Work out the finished part from the listing and answer in its coordinate system (mm). A direction names the side the tool comes from. Round coordinates to 2 decimals unless told otherwise and drop trailing zeros. Write each loop counter-clockwise with the first axis right and the second up, starting at its lowest first coordinate (ties: lowest second). Pieces come first, ordered by that corner, then holes. Notation, with made-up numbers: (20, 55.5) -> (61, 55.5) arc R27 ccw to (61, 90.5) -> close; hole circle Ø10 at (11, 48). An arc over 180 degrees is marked (long way). One line per item, written item: value.
```python
from build123d import *

# Parameters (mm, degrees)
RESSALTO_EXTRUS_O2_DEPTH = 25
ESBO_O9_R                = 3.75
ESBO_O9_R_2              = 1.65
CORTE_EXTRUS_O1_DEPTH    = 20
FILETE1_R                = 12.5
FILETE2_START            = -1
FILETE2_DEPTH            = 27
FILETE2_2_DEPTH          = 25
ESBO_O10_R               = 1
CORTE_EXTRUS_O2_DEPTH    = 82.160967921
ESBO_O11_R               = 7.5
CORTE_EXTRUS_O3_DEPTH    = 10
FILETE3_R                = 4


with BuildPart() as part:
    # Esboço2 → Ressalto-extrusão2 (new body)
    with BuildSketch(Plane(origin=(0, 0, 0), x_dir=(0, 0, -1), z_dir=(1, 0, 0))):
        Polygon((-5, 0), (0, 0), (5, 0), (69.5, -5.643018797), (69.5, -33.643018797), (67, -33.643018797), (67, -7.933846732), (4.890847643, -2.5), (0, -2.5), (-4.890847643, -2.5), (-67, -7.933846732), (-67, -33.643018797), (-69.5, -33.643018797), (-69.5, -5.643018797), align=None)
    extrude(amount=RESSALTO_EXTRUS_O2_DEPTH)

    # Esboço9 → Corte-extrusão1 (cut)
    with BuildSketch(Plane.XY.offset(69.5)):
        with Locations((12.5, -21.143018797)):
            Circle(ESBO_O9_R)
        with Locations((12.5, -12.643018797)):
            Circle(ESBO_O9_R_2)
        with Locations((21, -21.143018797)):
            Circle(ESBO_O9_R_2)
        with Locations((12.5, -29.643018797)):
            Circle(ESBO_O9_R_2)
        with Locations((4, -21.143018797)):
            Circle(ESBO_O9_R_2)
    corte_extrus_o1 = extrude(amount=-CORTE_EXTRUS_O1_DEPTH, mode=Mode.SUBTRACT)

    # Espelhar1: Corte-extrusão1 across plane
    add(corte_extrus_o1.mirror(Plane.XY), mode=Mode.SUBTRACT)

    # Filete1
    filete1_edges = [part.edges().sort_by_distance(p)[0] for p in [
        (0, -33.643018797, 68.25),
        (25, -33.643018797, 68.25),
        (25, -33.643018797, -68.25),
        (0, -33.643018797, -68.25),
    ]]
    fillet(filete1_edges, radius=FILETE1_R - 0.0001)  # a hair under: the kernel refuses the full size

    # Filete2: read off the stored shape, not the designer's step
    # Filete2 outline → Filete2 (cut)
    with BuildSketch(Plane.YZ.offset(FILETE2_START)):
        with BuildLine():
            Line((0, -5), (0, -4.912678114))
            ThreePointArc((0, -4.912678114), (-0.001903557, -4.999916889), (-0.007610604, -5.0869896))
            Line((-0.007610604, -5.0869896), (0, -5))
        make_face()
        with BuildLine():
            ThreePointArc((-7.475681145, 69.5), (-6.12450073, 68.974554674), (-5.483291749, 67.674311485))
            Line((-5.483291749, 67.674311485), (-5.643018797, 69.5))
            Line((-5.643018797, 69.5), (-7.475681145, 69.5))
        make_face()
        with BuildLine():
            ThreePointArc((-0.007610604, 5.0869896), (-0.001903557, 4.999916889), (0, 4.912678114))
            Line((0, 4.912678114), (0, 5))
            Line((0, 5), (-0.007610604, 5.0869896))
        make_face()
        with BuildLine():
            Line((-5.643018797, -69.5), (-5.483291749, -67.674311485))
            ThreePointArc((-5.483291749, -67.674311485), (-6.12450073, -68.974554674), (-7.475681145, -69.5))
            Line((-7.475681145, -69.5), (-5.643018797, -69.5))
        make_face()
    extrude(amount=FILETE2_DEPTH, mode=Mode.SUBTRACT)

    # Filete2 2 outline → Filete2 2 (add)
    with BuildSketch(Plane.YZ):
        with BuildLine():
            ThreePointArc((-9.766509081, 67), (-8.415328665, 66.474554674), (-7.774119684, 65.174311485))
            Line((-7.774119684, 65.174311485), (-7.933846732, 67))
            Line((-7.933846732, 67), (-9.766509081, 67))
        make_face()
        with BuildLine():
            ThreePointArc((-2.507610604, 4.977837242), (-2.501903557, 4.890764531), (-2.5, 4.803525757))
            Line((-2.5, 4.803525757), (-2.5, 4.890847643))
            Line((-2.5, 4.890847643), (-2.507610604, 4.977837242))
        make_face()
        with BuildLine():
            Line((-7.933846732, -67), (-7.774119684, -65.174311485))
            ThreePointArc((-7.774119684, -65.174311485), (-8.415328665, -66.474554674), (-9.766509081, -67))
            Line((-9.766509081, -67), (-7.933846732, -67))
        make_face()
        with BuildLine():
            ThreePointArc((-2.5, -4.803525757), (-2.501903557, -4.890764531), (-2.507610604, -4.977837242))
            Line((-2.507610604, -4.977837242), (-2.5, -4.890847643))
            Line((-2.5, -4.890847643), (-2.5, -4.803525757))
        make_face()
    extrude(amount=FILETE2_2_DEPTH)

    # Esboço10 → Corte-extrusão2 (cut, through all)
    with BuildSketch(Plane(origin=(0, 0, 0), x_dir=(1, 0, 0), z_dir=(0, 1, 0))):
        with Locations(Location((5, 0, 0), (0, 0, 270))):
            Circle(ESBO_O10_R)
        with Locations(Location((20, 0, 0), (0, 0, 270))):
            Circle(ESBO_O10_R)
    extrude(amount=-CORTE_EXTRUS_O2_DEPTH, mode=Mode.SUBTRACT)

    # Esboço11 → Corte-extrusão3 (cut, symmetric)
    with BuildSketch(Plane(origin=(0, 31.205699457, -34.0550451), x_dir=(1, 0, 0), z_dir=(0, -0.6755902076156625, 0.7372773368101221))):
        with Locations((-4.282064203, -51.1139893)):
            Circle(ESBO_O11_R)
        with Locations((29.282064203, -51.1139893)):
            Circle(ESBO_O11_R)
    corte_extrus_o3 = extrude(amount=CORTE_EXTRUS_O3_DEPTH, both=True, mode=Mode.SUBTRACT)

    # Espelhar2: Corte-extrusão3 across plane
    add(corte_extrus_o3.mirror(Plane.XY), mode=Mode.SUBTRACT)

    # Filete3
    filete3_edges = [part.edges().sort_by_distance(p)[0] for p in [
        (25, -15.140009882, -68.25),
        (25, -6.060544858, -59.930203155),
        (0, -6.060544858, -59.930203155),
        (0, -15.140009882, -68.25),
        (0, -15.140009882, 68.25),
        (0, -6.060544858, 59.930203155),
        (25, -15.140009882, 68.25),
        (25, -6.060544858, 59.930203155),
    ]]
    fillet(filete3_edges, radius=FILETE3_R)


solid = part.part
```
(1) Find section A-A on x = 17.5. Give the vertices of the cut face in (y, z), plus the area to 3 significant figures.
Reported:
outline: (-32.6, -69.5) -> (-7.48, -69.5) arc R2 ccw to (-5.48, -67.67) -> (-0.01, -5.09) arc R2 ccw to (0, -4.91) -> (0, 4.91) arc R2 ccw to (-0.01, 5.09) -> (-5.48, 67.67) arc R2 ccw to (-7.48, 69.5) -> (-32.6, 69.5) -> (-32.6, 67) -> (-9.77, 67) arc R2 cw to (-7.77, 65.17) -> (-2.51, 4.98) arc R2 cw to (-2.5, 4.8) -> (-2.5, -4.8) arc R2 cw to (-2.51, -4.98) -> (-7.77, -65.17) arc R2 cw to (-9.77, -67) -> (-32.6, -67) -> close
area: 472 mm2
(2) Find section B-B on z = -2.5. Give the vertices of the cut face in (x, y), plus the area to 3 significant figures.
Reported:
outline: (0, -2.5) -> (25, -2.5) -> (25, 0) -> (0, 0) -> close
area: 62.5 mm2
(3) Flat-ended cylindrical pins translate along their axes: pin 1 Ø2.5 at (x, y) = (12.5, -12.64) entering from +Z; pin 2 Ø5.5 at (x, y) = (21, -21.14) entering from -Z; pin 3 Ø7.5 at (x, z) = (16.5, -1.5) entering from -Y; pin 4 Ø1 at (x, z) = (20.5, 49) entering from -Y. Find the tip coordinate at first contact, or state that the pin passes through.
Reported:
pin 1: passes through
pin 2: stops at z = -69.5
pin 3: stops at y = -2.53
pin 4: stops at y = -6.4
(4) A tool of negligible diameter and unlimited length cuts with its end or side. For faces 1 (the face through (15, -18, 69.5)), 2 (the face through (15.1, -24.2, 67)), from which of +Z, -Z, +X, -X, +Y, -Y can it reach the whole face along a straight path? Write none if from no direction.
Reported:
face 1: +Z, +X, -X, +Y, -Y
face 2: +X, -X, -Y
(5) Consider probe 1 along X at (y, z) = (-1, 0); probe 2 along Z at (x, y) = (23.25, -14.5); probe 3 along Y at (x, z) = (21, -68). Determine where each line is inside the solid, lowest interval first.
Reported:
probe 1: x = 0 to 4, 6 to 19, 21 to 25
probe 2: z = -69.5 to -67, 67 to 69.5
probe 3: y = -30.31 to -22.79, -19.49 to -5.54
(6) For a pull along X with two mould halves and no side action, classify faces 3 (the face through (15, -17, -69.5)), 4 (the face through (9.52, -23.42, -68.27)), 5 (the face through (14.024, -13.275, 68.268)), 6 (the face through (21.44, -29.88, -68.23)) as pulls with the +X half, pulls with the -X half, needs draft (parallel to the pull), parting line crosses it, or undercut.
Reported:
face 3: needs draft
face 4: undercut
face 5: undercut
face 6: pulls with the +X half
(7) Find section C-C on z = 43.5. Give the vertices of the cut face in (x, y), plus the area to 3 significant figures.
Reported:
outline: (0, -5.88) -> (25, -5.88) -> (25, -3.37) -> (0, -3.37) -> close
area: 62.7 mm2
